Answer from the drawing. Dimensions are ordinates in mm from the lowest x, y and z of the part. A direction names the side the tool comes from. Give positions to 0.01 mm unless a question says otherwise; leave off trailing zeros. Write each loop counter-clockwise with the first axis right and the second up, starting at its lowest first coordinate (ties: lowest second). Pieces come first, ordered by that corner, then holes.
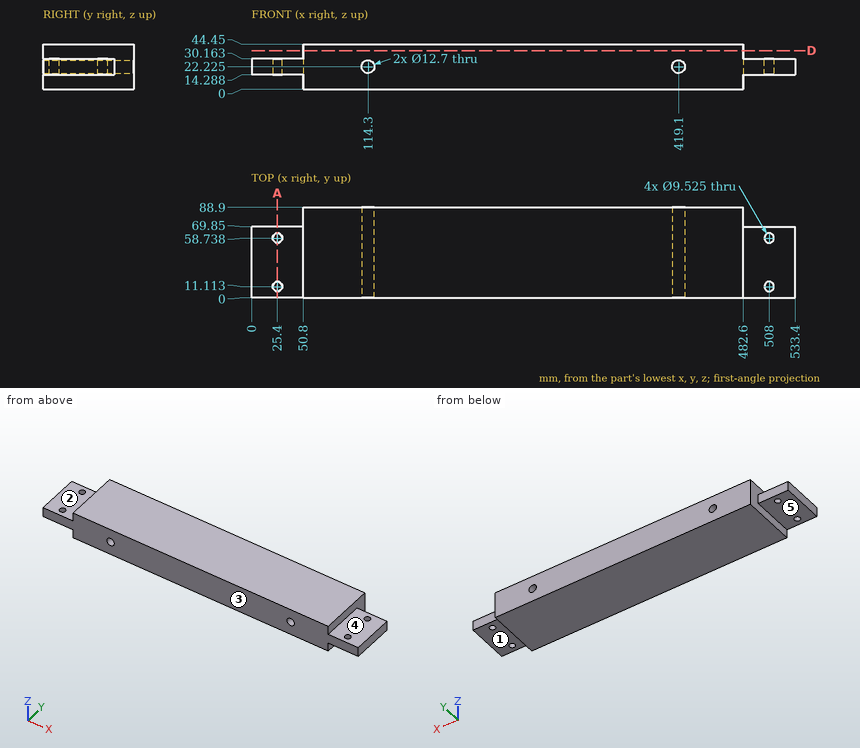
Item 1: Which of the six approach directions +Z, -Z, +X, -X, +Y, -Y give full straight-line access (tool end or side, diameter ignored) to the marked faces 1, 2, 3, 4 and 5?
Conclusion:
face 1: -Z, +X, +Y, -Y
face 2: +Z, -X, +Y, -Y
face 3: +Z, -Z, +X, -X, -Y
face 4: +Z, +X, +Y, -Y
face 5: -Z, -X, +Y, -Y
Item 2: Each of these flat-tipped pins is pushed along its axis until it touches: P1, Ø7.5, axis at x = 25.4, y = 58.74, coming from the -Z side; P2, Ø5, axis at x = 503, z = 18.5, coming from the +Y side; P3, Ø12, axis at x = 408, y = 36.5, coming from the -Z side; P4, Ø3, axis at y = 36, z = 33, coming from the +X side. Where does it stop, or does it pass through?
Conclusion:
P1: passes through
P2: stops at y = 69.85
P3: stops at z = 0
P4: stops at x = 482.6
Item 3: A cutting plane is placed at A-A, the plane x = 25.4. Count the separate pieces of the cut face and the enclosed holes in it.
Conclusion:
separate pieces: 3
enclosed holes: 0
Item 4: Consider probe 1 along X at (y, z) = (64.5, 37); probe 2 along Y at (x, z) = (496.5, 15); probe 3 along Z at (x, y) = (503.5, 26.5). Determine where each line is inside the solid, lowest interval first.
Conclusion:
probe 1: x = 50.8 to 482.6
probe 2: y = 0 to 69.85
probe 3: z = 14.29 to 30.16
Item 5: A cutting plane is placed at D-D, the plane z = 38. Give the vertices of the cut face in (x, y), plus the area to 3 significant figures.
Conclusion:
outline: (50.8, 0) - (482.6, 0) - (482.6, 88.9) - (50.8, 88.9) - close
area: 38,400 mm2
